Here's how the part is built. I have some questions about the finished solid (model axes, mm). A direction names the side the tool comes from. Round coordinates to 2 decimals unless told otherwise and drop trailing zeros. Write each loop counter-clockwise with the first axis right and the second up, starting at its lowest first coordinate (ties: lowest second). Pieces come first, ordered by that corner, then holes. Notation, with made-up numbers: (-21.75, -8.5) -> (-7.75, -8.5) arc R34 ccw to (-7.75, 21.5) -> close; hole circle Ø8 at (-2, 18.5). An arc over 180 degrees is marked (long way). Put each result on its own line as item: value. Start each with the question number.
1) I want a section at B-B, the plane x = 0. List the corners of the cut face in (y, z) for me.
2) We'd pull the mould along Z, two halves only. Please class faces 1 (the flat face through (-14, 70.083, 23)), 2 (the conical face through (-7.885, 31.054, 2.483)), 3 (the cylindrical face through (-5, 23.4, 1.6)): released by +Z, released by -Z, zero draft, split by the parting line, or undercut.
3) If I drill on line 1 along Z through (x, y) = (0, 61.75); line 2 along Z through (x, y) = (0, 25.5), over which ranges is the centre line in solid material (lowest first)? Write a range as [from, to].
4) I want a section at C-C, the plane y = 26. List the corners of the cut face in (x, z) for me.
5) Which directions (+Z, -Z, +X, -X, +Y, -Y) give clear straight access to the entire face, cutting with the end or side of a thin tool? Please do faces 4 (the cylindrical face through (-13.01, 59.7, -25.02)), 5 (the cylindrical face through (-3.35, 22.73, -6.43)), 6 (the cylindrical face through (3.411, 60.392, 25.977)).
6) I want a section at A-A, the plane z = 0. List the corners of the cut face in (x, y) for me, then the cut area to 3 significant figures.
7) Will these pins go through, and if not, where does the flat tip stop? P1, Ø1.5, axis at x = 12, z = 9, coming from the -Y side; P2, Ø6.5, axis at x = 0, z = 0, coming from the -Y side; P3, Ø1, axis at x = -15.5, z = 7.5, coming from the -Y side; P4, Ø8, axis at x = 0, z = -19, coming from the -Y side.
from build123d import *

# Parameters (mm, degrees)
FILLET1_R = 0.5


with BuildPart() as part:
    # Sketch1 → Revolve1 (revolve)
    with BuildSketch(Plane.XY):
        Polygon((-5.25, 15.08330694), (-5.25, 30.939040938), (-26.2, 50.939040938), (-26.2, 70.08330694), (-28.2, 70.08330694), (-28.2, 50.08330694), (-7.25, 30.08330694), (-7.25, 15.08330694), align=None)
    revolve(axis=Axis((0, 0, 0), (0, 1, 0)))

    # Fillet1
    fillet1_edges = [part.edges().sort_by_distance(p)[0] for p in [
        (7.25, 15.08330694, 0),
        (28.2, 70.08330694, 0),
        (26.2, 70.08330694, 0),
        (5.25, 15.08330694, 0),
    ]]
    fillet(fillet1_edges, radius=FILLET1_R)


solid = part.part
Findings:
1. outline: (15.08, -6.75) arc R0.5 ccw to (15.58, -7.25) -> (30.08, -7.25) -> (50.08, -28.2) -> (69.58, -28.2) arc R0.5 ccw to (70.08, -27.7) -> (70.08, -26.7) arc R0.5 ccw to (69.58, -26.2) -> (50.94, -26.2) -> (30.94, -5.25) -> (15.58, -5.25) arc R0.5 ccw to (15.08, -5.75) -> close; (15.08, 5.75) arc R0.5 ccw to (15.58, 5.25) -> (30.94, 5.25) -> (50.94, 26.2) -> (69.58, 26.2) arc R0.5 ccw to (70.08, 26.7) -> (70.08, 27.7) arc R0.5 ccw to (69.58, 28.2) -> (50.08, 28.2) -> (30.08, 7.25) -> (15.58, 7.25) arc R0.5 ccw to (15.08, 6.75) -> close
2. face 1: zero draft
2. face 2: split by the parting line
2. face 3: undercut
3. line 1: z = [-28.2, -26.2], [26.2, 28.2]
3. line 2: z = [-7.25, -5.25], [5.25, 7.25]
4. outline: circle Ø14.5 at (0, 0); hole circle Ø10.5 at (0, 0)
5. face 4: +Y, -Y
5. face 5: -Y
5. face 6: +Y
6. outline: (-28.2, 50.08) -> (-7.25, 30.08) -> (-7.25, 15.58) arc R0.5 ccw to (-6.75, 15.08) -> (-5.75, 15.08) arc R0.5 ccw to (-5.25, 15.58) -> (-5.25, 30.94) -> (-26.2, 50.94) -> (-26.2, 69.58) arc R0.5 ccw to (-26.7, 70.08) -> (-27.7, 70.08) arc R0.5 ccw to (-28.2, 69.58) -> close; (5.25, 15.58) arc R0.5 ccw to (5.75, 15.08) -> (6.75, 15.08) arc R0.5 ccw to (7.25, 15.58) -> (7.25, 30.08) -> (28.2, 50.08) -> (28.2, 69.58) arc R0.5 ccw to (27.7, 70.08) -> (26.7, 70.08) arc R0.5 ccw to (26.2, 69.58) -> (26.2, 50.94) -> (5.25, 30.94) -> close
6. area: 255 mm2
7. P1: stops at y = 36.77
7. P2: passes through
7. P3: stops at y = 39.12
7. P4: stops at y = 37.48
